from build123d import *

# Parameters (mm, degrees)
SKETCH1_W           = 51
SKETCH1_H           = 80
SKETCH1_R           = 1.7
BOSS_EXTRUDE1_DEPTH = 10
SKETCH2_R           = 7.525
CUT_EXTRUDE1_DEPTH  = 45.2
SKETCH3_R           = 4.5
CUT_EXTRUDE2_DEPTH  = 96.399161422
SKETCH4_R           = 3
CUT_EXTRUDE3_DEPTH  = 3


with BuildPart() as part:
    # Sketch1 → Boss-Extrude1 (new body)
    with BuildSketch(Plane.XY):
        with Locations((25.5, 40)):
            Rectangle(SKETCH1_W, SKETCH1_H)
        with Locations((7, 55)):
            Circle(SKETCH1_R, mode=Mode.SUBTRACT)
        with Locations((44, 55)):
            Circle(SKETCH1_R, mode=Mode.SUBTRACT)
        with Locations((7, 25)):
            Circle(SKETCH1_R, mode=Mode.SUBTRACT)
        with Locations((44, 25)):
            Circle(SKETCH1_R, mode=Mode.SUBTRACT)
    extrude(amount=BOSS_EXTRUDE1_DEPTH)

    # Sketch2 → Cut-Extrude1 (cut)
    with BuildSketch(Plane.ZY.offset(-3)):
        with Locations((10, 71)):
            Circle(SKETCH2_R)
        with Locations((10, 9)):
            Circle(SKETCH2_R)
    extrude(amount=-CUT_EXTRUDE1_DEPTH, mode=Mode.SUBTRACT)

    # Sketch3 → Cut-Extrude2 (cut, through all)
    with BuildSketch(Plane.ZY):
        with Locations((10, 71)):
            Circle(SKETCH3_R)
        with Locations((10, 9)):
            Circle(SKETCH3_R)
    extrude(amount=-CUT_EXTRUDE2_DEPTH, mode=Mode.SUBTRACT)

    # Sketch4 → Cut-Extrude3 (cut)
    with BuildSketch(Plane(origin=(0, 0, 0), x_dir=(-1, 0, 0), z_dir=(0, 0, -1))):
        with Locations((-44, 55)):
            Circle(SKETCH4_R)
        with Locations((-7, 55)):
            Circle(SKETCH4_R)
        with Locations((-7, 25)):
            Circle(SKETCH4_R)
        with Locations((-44, 25)):
            Circle(SKETCH4_R)
    extrude(amount=-CUT_EXTRUDE3_DEPTH, mode=Mode.SUBTRACT)


solid = part.part
Could you check a few things on this model? Use its own coordinates, in mm. A direction names the side the tool comes from. Give positions to 0.01 mm unless a question says otherwise; leave off trailing zeros. Order: outer loops, then holes, each group sorted by start corner. A loop starts at its lowest first (then second) coordinate and runs counter-clockwise, first axis right, second up.
Item 1: For faces 4 (the face through (42.75, 26.15, 6.45)), 5 (the face through (3, 9, 5)), 6 (the face through (7, 58, 1)), which set-ups out of +Z, -Z, +X, -X, +Y, -Y let a thin tool reach every point of the face, with its end or its side?
Item 2: If we section it at B-B, the plane x = 7: Write out the boundary of the cut face in (y, z) (3 decimals), plus the area to 3 significant figures.
Item 3: If we section it at A-A, the plane y = 55: Write out the boundary of the cut face in (x, z), plus the area to 3 significant figures.
Item 4: If we mould it in two halves opening along Y, with no side actions, what happens to faces 1 (the face through (49.6, 9.1, 5.5)), 2 (the face through (25, 0, 5)), 3 (the face through (0, 39, 5))? For each: pulls with the +Y half, pulls with the -Y half, needs draft (parallel to the pull), parting line crosses it, or undercut.
Item 5: I'm going to push a flat-ended pin straight in: pin 1 (5.5 mm diameter, centred on x = 44, y = 25, fed in from -Z). Where does the tip first touch, or does it pass through?
Item 6: If we section it at D-D, the plane y = 71: Write out the boundary of the cut face in (x, z) (3 decimals).
Item 7: I need wall thicknesses on line 1 (X direction, y = 25, z = 7.75); line 2 (Y direction, x = 26.5, z = 8.5); line 3 (X direction, y = 54, z = 2.5). Which ranges of each line are inside material? Lowest first, please.
Item 8: If we section it at C-C, the plane z = 8.5: Count the separate pieces of the cut face and the enclosed holes in it, plus the area to 3 significant figures.
Values:
1. face 4: +Z, -Z
1. face 5: +Z
1. face 6: -Z
2. outline: (0, 0) - (22, 0) - (22, 3) - (23.3, 3) - (23.3, 10) - (16.525, 10) arc R7.525 cw to (1.475, 10) - (0, 10) - close; (26.7, 3) - (28, 3) - (28, 0) - (52, 0) - (52, 3) - (53.3, 3) - (53.3, 10) - (26.7, 10) - close; (56.7, 3) - (58, 3) - (58, 0) - (80, 0) - (80, 10) - (78.525, 10) arc R7.525 cw to (63.475, 10) - (56.7, 10) - close
2. area: 539 mm2
3. outline: (0, 0) - (4, 0) - (4, 3) - (5.3, 3) - (5.3, 10) - (0, 10) - close; (8.7, 3) - (10, 3) - (10, 0) - (41, 0) - (41, 3) - (42.3, 3) - (42.3, 10) - (8.7, 10) - close; (45.7, 3) - (47, 3) - (47, 0) - (51, 0) - (51, 10) - (45.7, 10) - close
3. area: 426 mm2
4. face 1: undercut
4. face 2: pulls with the -Y half
4. face 3: needs draft
5. pin 1: stops at z = 3
6. outline: (0, 0) - (51, 0) - (51, 5.5) - (48.2, 5.5) - (48.2, 2.475) - (3, 2.475) - (3, 5.5) - (0, 5.5) - close
7. line 1: x = 0 to 5.3, 8.7 to 42.3, 45.7 to 51
7. line 2: y = 0 to 1.63, 16.37 to 63.63, 78.37 to 80
7. line 3: x = 0 to 4.17, 9.83 to 41.17, 46.83 to 51
8. separate pieces: 3
8. enclosed holes: 4
8. area: 2,610 mm2
